Autodesk Fusion 360 part; units mm, degrees
sketch "Sketch1" plane through (0, 0, 0) normal (1, 0, 0) x (0, 1, 0)
  line L0 (6.4, 0) -> (6.4, 25)
  line L1 (0, 25) -> (0, 0)
  line L2 (6.4, 0.1899) -> (6.4, 25)
  line L3 (0, 0) -> (18, 0)
  line L4 (0, 1) -> (0, 0)
  line L5 (6.4, 25) -> (7.4, 25)
  line L6 (18, 0) -> (18, 1)
  line L7 (18, 1) -> (16.5, 1) construction
  line L8 (7.4, 25) -> (8.4, 25)
  line L9 (18, 1) -> (18, 2)
  arc A0 (8.4, 25) -> (18, 2) centre (37.363, 23.5854) ccw
  line L10 (8.4, 25) -> (8.4, 7)
  line L11 (18, 2) -> (9, 2)
  line L12 (18, 2) -> (16, 2)
  arc A1 (8.4, 14.3286) -> (16, 2) centre (36.7237, 23.282) ccw
  line L13 (8.4, 7) -> (8.4, 2)
  line L14 (8.4, 2) -> (9, 2)
  arc A2 (8.4, 4.5) -> (10.5136, 2) centre (10.9353, 4.5) ccw
  dimension "d1" = 6.4
  dimension "d2" = 25
  dimension "d10" = 1
  dimension "d11" = 1
  dimension "d14" = 1
  dimension "d15" = 1
  dimension "d16" = 2
revolve "Revolve3" add sketch "Sketch1" angle 360 about axis through (0, 0, 25) along (0, 0, -1) contours L0 L2 L3 L5 L6 L8 L9 A0 L10 L11 L12 L13 L14 | A0 L10 L11 L12 A1 | L11 L13 L14 A2
chamfer "Chamfer4" distance 0.75 angle 45 1 edges at (-16.7819, 6.5091, 2)
chamfer "Chamfer5" distance 0.5 angle 45 1 edges at (-5.9669, 2.3143, 0)
fillet "Fillet1" radius 1 1 edges at (-7.8315, 3.0376, 25)
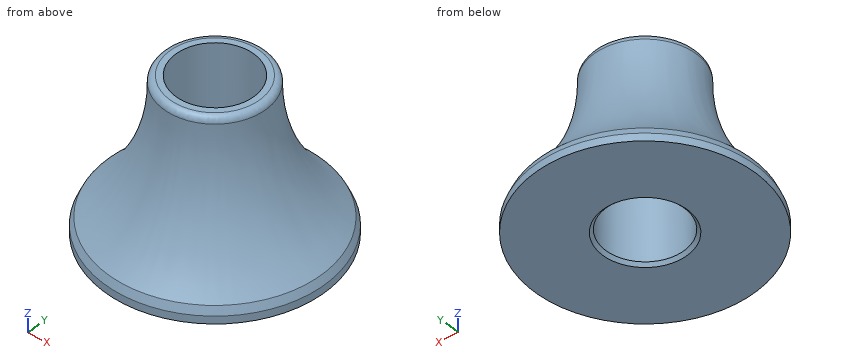
The listing builds one solid part. Answer for the finished solid, in the listing's coordinates (mm). Coordinates: 2 decimals unless noted, no trailing zeros. Loops run counter-clockwise (first coordinate to the right, second up) from the corner with the lowest first, then second, coordinate; pieces in that order, holes last. Notation, with made-up numbers: (-13.5, 57.25) - (0.5, 57.25) arc R19 ccw to (0.5, 90.25) - close; hole circle Ø10 at (73, -36.5). An arc over 180 degrees is marked (long way). Use a Markdown table: item, result. Add a question column.
1) The part is cut by section B-B, the plane y = 2.5. State how many separate pieces and enclosed holes the cut face has, and give its area (3 significant figures).
2) Given pin 1 (1.5 mm diameter, centred on y = -6.5, z = 19.5, fed in from -X); pin 2 (6 mm diameter, centred on y = -2.5, z = 7.5, fed in from +X); pin 3 (1.5 mm diameter, centred on x = -8, z = 3.5, fed in from -Y); pin 4 (10 mm diameter, centred on x = 0, y = 0, fed in from +Z), each flat-ended and moving along its own axis, determine where each tip first touches the part or whether it passes through.
3) Find the intervals of material crossed by line 1 (X direction, y = -2, z = 12.5); line 2 (Y direction, x = 3, z = 11); line 3 (X direction, y = 4, z = 2.25), in increasing order.
4) The part is cut by section D-D, the plane z = 22.75. Give the vertices of the cut face in (x, y), and give its area (3 significant figures).
5) The part is cut by section A-A, the plane z = 3.5. Give the vertices of the cut face in (x, y).
Here are the results:
| question | item | result |
|---|---|---|
| 1 | separate pieces | 2 |
| 1 | enclosed holes | 2 |
| 1 | area | 198 mm^2 |
| 2 | pin 1 | stops at x = -6.48 |
| 2 | pin 2 | stops at x = 15.37 |
| 2 | pin 3 | stops at y = -15.3 |
| 2 | pin 4 | passes through |
| 3 | line 1 | x = -10.38 to -8.82, -8.16 to -6.08, 6.08 to 8.16, 8.82 to 10.38 |
| 3 | line 2 | y = -10.83 to -9.2, -7.85 to -5.65, 5.65 to 7.85, 9.2 to 10.83 |
| 3 | line 3 | x = -17.1 to -15.23, -8.91 to -5, 5 to 8.91, 15.23 to 17.1 |
| 4 | outline | circle Ø16.76 at (0, 0); hole circle Ø12.8 at (0, 0) |
| 4 | area | 91.8 mm^2 |
| 5 | outline | circle Ø32.9 at (0, 0); circle Ø17.21 at (0, 0); hole circle Ø29.13 at (0, 0); hole circle Ø12.8 at (0, 0) |
